from build123d import *

# Parameters (mm, degrees)
RESSALTO_EXTRUS_O1_DEPTH = 2
FILETE1_R                = 10


with BuildPart() as part:
    # Esboço1 → Ressalto-extrusão1 (new body)
    with BuildSketch(Plane(origin=(0, 0, 0), x_dir=(1, 0, 0), z_dir=(0, 1, 0))):
        Polygon((0, 0), (70, 0), (70, 70), (24.544299076, 49.952139866), align=None)
    extrude(amount=RESSALTO_EXTRUS_O1_DEPTH)

    # Filete1
    filete1_edges = [part.edges().sort_by_distance(p)[0] for p in [
        (24.544299076, 1, -49.952139866),
    ]]
    fillet(filete1_edges, radius=FILETE1_R)


solid = part.part
Read the model definition and answer for the solid it produces. Units are mm, in the model's axes. Round coordinates to 2 decimals unless told otherwise and drop trailing zeros. Write each loop counter-clockwise with the first axis right and the second up, starting at its lowest first coordinate (ties: lowest second). Pieces come first, ordered by that corner, then holes.
1. The part is cut by section A-A, the plane y = 0.6. Determine the outline of the cut face in (x, z), then the cut area to 3 significant figures.
2. The part is cut by section C-C, the plane z = -61. Determine the outline of the cut face in (x, y).
3. Given pin 1 Ø1 at (x, y) = (34, 1.5) entering from -Z; pin 2 Ø1 at (y, z) = (2, -31.5) entering from -X, each flat-ended and moving along its own axis, determine where each tip first touches the part or whether it passes through.
4. The part is cut by section B-B, the plane x = 6. Determine the outline of the cut face in (y, z), then the cut area to 3 significant figures.
5. Straight lines are drawn through the part: L1, parallel to Z at x = 27.5, y = 0.1; L2, parallel to Z at x = 31, y = 0.55; L3, parallel to X at y = 1.65, z = -65.5. For each, find the intervals that lie inside material, in ascending order.
Values:
1. outline: (0, 0) - (22.94, -46.68) arc R10 ccw to (27.88, -51.42) - (70, -70) - (70, 0) - close
1. area: 3,340 mm2
2. outline: (49.59, 0) - (70, 0) - (70, 2) - (49.59, 2) - close
3. pin 1: stops at z = -54.34
3. pin 2: stops at x = 15.23
4. outline: (0, -12.21) - (2, -12.21) - (2, 0) - (0, 0) - close
4. area: 24.4 mm2
5. L1: z = -51.25 to 0
5. L2: z = -52.8 to 0
5. L3: x = 59.8 to 70
